Input: dimensioned drawing with shaded views. Units: mm. Origin: part minimum x, y, z. Give positions to 0.01 mm unless a question says otherwise; leave off trailing zeros. Loops run counter-clockwise (first coordinate to the right, second up) from the corner with the lowest first, then second, coordinate; pieces in that order, holes last. Notation, with made-up numbers: (-4.75, 84) -> (1.25, 84) arc R15 cw to (1.25, 93) -> close; hole circle Ø6 at (-31, 77). An arc over 180 degrees is marked (long way). Answer as a JSON object with one key per item and string values.
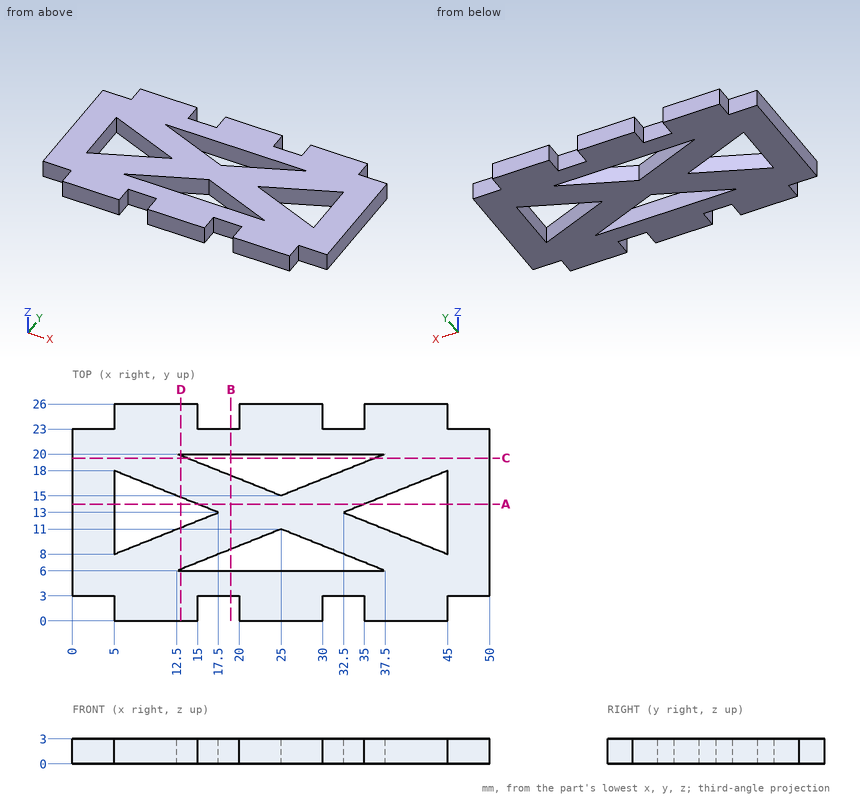
Q1. Ray query, line 1 along X through (y, z) = (23.75, 1.45); line 2 along Y through (x, z) = (31, 2); line 3 along Y through (x, z) = (32, 1.1). Return the intervals inside material, ascending.
Evaluation:
{"line 1": "x = 5 to 15, 20 to 30, 35 to 45", "line 2": "y = 3 to 6, 8.6 to 17.4, 20 to 23", "line 3": "y = 3 to 6, 8.2 to 17.8, 20 to 23"}
Q2. Section C-C, the plane y = 19.5. Return the cut outline in (x, z).
Evaluation:
{"outline": "(0, 0) -> (13.75, 0) -> (13.75, 3) -> (0, 3) -> close; (36.25, 0) -> (50, 0) -> (50, 3) -> (36.25, 3) -> close"}
Q3. Section D-D, the plane x = 13. Return the cut outline in (y, z), then the cut area to 3 significant figures.
Evaluation:
{"outline": "(0, 0) -> (6, 0) -> (6, 3) -> (0, 3) -> close; (6.2, 0) -> (11.2, 0) -> (11.2, 3) -> (6.2, 3) -> close; (14.8, 0) -> (19.8, 0) -> (19.8, 3) -> (14.8, 3) -> close; (20, 0) -> (26, 0) -> (26, 3) -> (20, 3) -> close", "area": "66.0 mm2"}
Q4. Pin query (flat end, axial travel): pin 1 (1.5 mm diameter, centred on x = 46.5, z = 2, fed in from +Y); pin 2 (0.9 mm diameter, centred on y = 25, z = 1, fed in from +X); pin 3 (1.5 mm diameter, centred on y = 1, z = 1, fed in from -X); pin 4 (1.5 mm diameter, centred on x = 21.5, y = 18, fed in from -Z). Return the tip coordinate at first contact, or that it passes through.
Evaluation:
{"pin 1": "stops at y = 23", "pin 2": "stops at x = 45", "pin 3": "stops at x = 5", "pin 4": "passes through"}
Q5. Section A-A, the plane y = 14. Return the cut outline in (x, z).
Evaluation:
{"outline": "(0, 0) -> (5, 0) -> (5, 3) -> (0, 3) -> close; (15, 0) -> (35, 0) -> (35, 3) -> (15, 3) -> close; (45, 0) -> (50, 0) -> (50, 3) -> (45, 3) -> close"}
Q6. Section B-B, the plane x = 19. Return the cut outline in (y, z), then the cut area to 3 significant figures.
Evaluation:
{"outline": "(3, 0) -> (6, 0) -> (6, 3) -> (3, 3) -> close; (8.6, 0) -> (17.4, 0) -> (17.4, 3) -> (8.6, 3) -> close; (20, 0) -> (23, 0) -> (23, 3) -> (20, 3) -> close", "area": "44.4 mm2"}
